Could you check a few things on this model? Use its own coordinates, in mm. Face numbers are marked on the shaded views. A direction names the side the tool comes from. Give positions to 0.01 mm unless a question says otherwise; leave off trailing zeros. Loops run counter-clockwise (first coordinate to the right, second up) from the corner with the lowest first, then second, coordinate; pieces in that order, holes last. Notation, with made-up numbers: (24, 44.25) - (78, 44.25) arc R28 cw to (78, 82.25) - close; hole circle Ø10 at (7.25, 61). An arc over 180 degrees is marked (long way). Write each question's results on one line, items separated by ' | '. Start each with the question number.
(1) On a 3-axis mill with a long thin cutter (end or side, diameter ignored), from which of +Z, -Z, +X, -X, +Y, -Y can I reach the whole of each face in a straight line? I mean the marked faces 1 and 2. Say none if no direction works.
(2) Suppose I cut it at A-A (z = 24). Please give me the cut outline in (x, y), and give its area (3 significant figures).
(3) Suppose I cut it at B-B (x = 55). Please give me the cut outline in (y, z).
(4) For pin 1 (1.5 mm diameter, centred on x = 53, z = 1, fed in from +Y); pin 2 (4 mm diameter, centred on x = 30, y = 25, fed in from -Z) (3 decimals); pin 3 (1 mm diameter, centred on x = 54, y = 6.5, fed in from +Z); pin 4 (1.5 mm diameter, centred on y = 37.5, z = 2, fed in from +X), each with a flat end and sliding along its axis, tell me the tip position at first contact or that it passes through.
(5) Suppose I cut it at C-C (y = 5). Please give me the cut outline in (x, z), and give its area (3 significant figures).
(6) Suppose I cut it at D-D (x = 10). Please give me the cut outline in (y, z).
(7) I need wall thicknesses on line 1 (Y direction, x = 10, z = 0.85); line 2 (Z direction, x = 20, y = 22). Which ranges of each line are inside material? Lowest first, please.
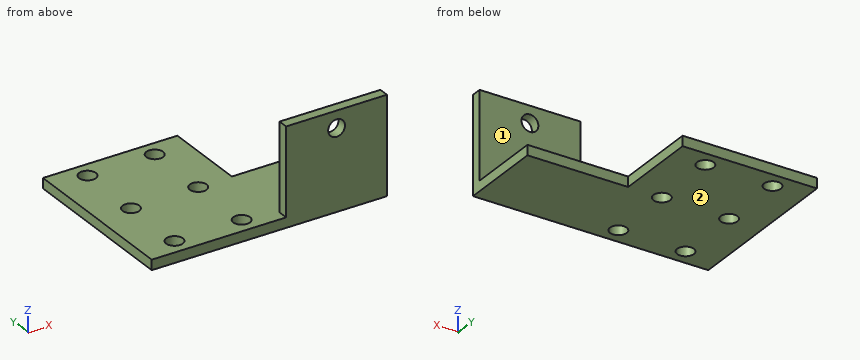
from build123d import *

# Parameters (mm, degrees)
SKETCH1_W               = 40
SKETCH1_H               = 50
SKETCH1_R               = 2.5
BOSS_EXTRUDE1_DEPTH     = 3
BOSS_EXTRUDE2_DEPTH     = 30
SKETCH4_R               = 2.5
CUT_EXTRUDE2_DEPTH      = 48
CUT_EXTRUDE2_DEPTH_BACK = 4


with BuildPart() as part:
    # Sketch1 → Boss-Extrude1 (new body)
    with BuildSketch(Plane.XY):
        with Locations((20, 25)):
            Rectangle(SKETCH1_W, SKETCH1_H)
        with Locations((30, 45)):
            Circle(SKETCH1_R, mode=Mode.SUBTRACT)
        with Locations((10, 45)):
            Circle(SKETCH1_R, mode=Mode.SUBTRACT)
        with Locations((10, 25)):
            Circle(SKETCH1_R, mode=Mode.SUBTRACT)
        with Locations((10, 5)):
            Circle(SKETCH1_R, mode=Mode.SUBTRACT)
        with Locations((30, 25)):
            Circle(SKETCH1_R, mode=Mode.SUBTRACT)
        with Locations((30, 5)):
            Circle(SKETCH1_R, mode=Mode.SUBTRACT)
    extrude(amount=BOSS_EXTRUDE1_DEPTH)

    # Sketch2 → Boss-Extrude2 (add)
    with BuildSketch(Plane(origin=(40, 0, 0), x_dir=(0, 0, -1), z_dir=(1, 0, 0))):
        Polygon((0, 0), (-29, 0), (-29, 3), (-3, 3), (-3, 25), (0, 25), align=None)
    extrude(amount=BOSS_EXTRUDE2_DEPTH)

    # Sketch4 → Cut-Extrude2 (cut, two sides)
    with BuildSketch(Plane(origin=(0, 3, 0), x_dir=(1, 0, 0), z_dir=(0, 1, 0))) as cut_extrude2_sk:
        with Locations((55, -24)):
            Circle(SKETCH4_R)
    extrude(amount=CUT_EXTRUDE2_DEPTH, mode=Mode.SUBTRACT)
    extrude(cut_extrude2_sk.sketch, amount=-CUT_EXTRUDE2_DEPTH_BACK, mode=Mode.SUBTRACT)


solid = part.part
Output values:
1) face 1: +Z, +X, -X, +Y | face 2: -Z, +X, -X, +Y, -Y
2) outline: (40, 0) - (52.5, 0) - (52.5, 3) - (40, 3) - close; (57.5, 0) - (70, 0) - (70, 3) - (57.5, 3) - close | area: 75.0 mm2
3) outline: (0, 0) - (25, 0) - (25, 3) - (3, 3) - (3, 21.5) - (0, 21.5) - close; (0, 26.5) - (3, 26.5) - (3, 29) - (0, 29) - close
4) pin 1: y = 25 | pin 2: through | pin 3: z = 3 | pin 4: x = 40
5) outline: (0, 0) - (7.5, 0) - (7.5, 3) - (0, 3) - close; (12.5, 0) - (27.5, 0) - (27.5, 3) - (12.5, 3) - close; (32.5, 0) - (70, 0) - (70, 3) - (32.5, 3) - close | area: 180 mm2
6) outline: (0, 0) - (2.5, 0) - (2.5, 3) - (0, 3) - close; (7.5, 0) - (22.5, 0) - (22.5, 3) - (7.5, 3) - close; (27.5, 0) - (42.5, 0) - (42.5, 3) - (27.5, 3) - close; (47.5, 0) - (50, 0) - (50, 3) - (47.5, 3) - close
7) line 1: 0 to 2.5, 7.5 to 22.5, 27.5 to 42.5, 47.5 to 50 | line 2: 0 to 3
